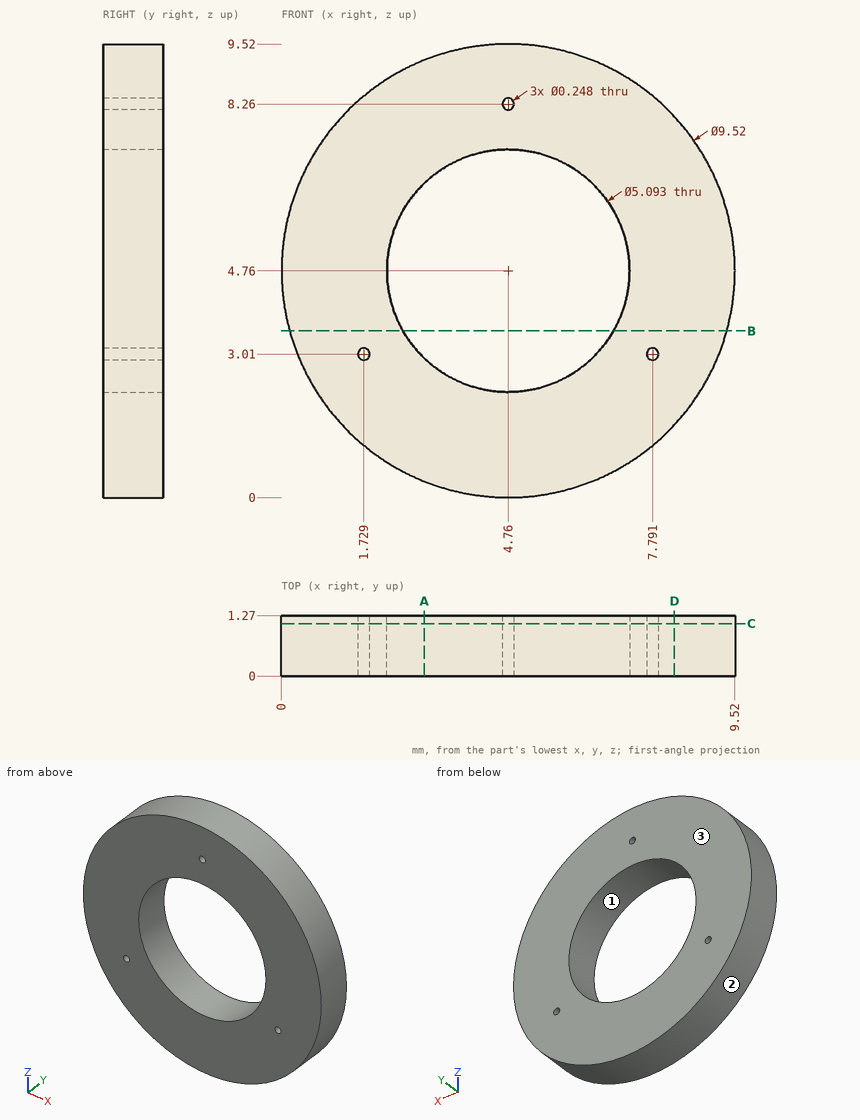
Verification items for this drawing (mm, ordinates from the low corner). Coordinates: 2 decimals unless noted, no trailing zeros. Order: outer loops, then holes, each group sorted by start corner. A loop starts at its lowest first (then second) coordinate and runs counter-clockwise, first axis right, second up. Notation, with made-up numbers: (-37.5, 2) - (-33.5, 2) arc R14 cw to (-33.5, 28) - close; hole circle Ø3 at (10, 87.25). An arc over 180 degrees is marked (long way). Use one line per item in the form item = value.
1. Section check A-A (x = 3). Record the boundary of the cut face in (y, z).
Here are the results:
outline = (0, 0.34) - (1.27, 0.34) - (1.27, 2.92) - (0, 2.92) - close; (0, 6.6) - (1.27, 6.6) - (1.27, 9.18) - (0, 9.18) - close
2. Draft check along X on the marked faces 1, 2 and 3. Enter one of: pulls with the +X half, pulls with the -X half, needs draft (parallel to the pull), parting line crosses it, or undercut.
Here are the results:
face_1 = undercut
face_2 = parting line crosses it
face_3 = needs draft
3. Scan lines: line 1 (Z direction, x = 6, y = 0.55) (1 decimal); line 2 (X direction, y = 0.25, z = 5.25) (1 decimal); line 3 (X direction, y = 0.95, z = 5) (1 decimal). Record each from-to range of solid material in increasing order.
Here are the results:
line_1 = 0.2 to 2.5, 7 to 9.4
line_2 = 0 to 2.3, 7.3 to 9.5
line_3 = 0 to 2.2, 7.3 to 9.5
4. Section check D-D (x = 8.25). Record the boundary of the cut face in (y, z).
Here are the results:
outline = (0, 1.52) - (1.27, 1.52) - (1.27, 8) - (0, 8) - close
5. Section check B-B (z = 3.5). Record the boundary of the cut face in (x, y).
Here are the results:
outline = (0.17, 0) - (2.55, 0) - (2.55, 1.27) - (0.17, 1.27) - close; (6.97, 0) - (9.35, 0) - (9.35, 1.27) - (6.97, 1.27) - close
6. Section check C-C (y = 1.1). Record the boundary of the cut face in (x, z) (1 decimal).
Here are the results:
outline = circle Ø9.5 at (4.8, 4.8); hole circle Ø0.2 at (1.7, 3); hole circle Ø5.1 at (4.8, 4.8); hole circle Ø0.2 at (4.8, 8.3); hole circle Ø0.2 at (7.8, 3)
